Autodesk Inventor part; units mm, degrees
ref_plane "to_body_XY" through (0, 0, 0) normal (0, 1, 0) x (1, 0, 0)
ref_plane "to_body_YZ" through (0, 0, 0) normal (1, 0, 0) x (0, 0, -1)
ref_plane "to_body_ZX" through (0, 0, 0) normal (0, 0, -1) x (0, 1, 0)
sketch "Sketch_1" plane through (0, 0, 0) normal (0, 1, 0) x (-1, 0, 0)
  line L0 (3.9497, -6.3754) -> (3.9497, 6.3754)
  arc A0 (3.9497, 6.3754) -> (3.8227, 6.5024) centre (3.8227, 6.3754) ccw
  line L1 (3.8227, 6.5024) -> (-3.8227, 6.5024)
  arc A1 (-3.8227, 6.5024) -> (-3.9497, 6.3754) centre (-3.8227, 6.3754) ccw
  line L2 (-3.9497, 6.3754) -> (-3.9497, -6.3754)
  arc A2 (-3.9497, -6.3754) -> (-3.8227, -6.5024) centre (-3.8227, -6.3754) ccw
  line L3 (-3.8227, -6.5024) -> (3.8227, -6.5024)
  arc A3 (3.8227, -6.5024) -> (3.9497, -6.3754) centre (3.8227, -6.3754) ccw
  line L4 (3.6957, -6.2484) -> (3.6957, 6.2484)
  line L5 (3.6957, 6.2484) -> (-3.6957, 6.2484)
  line L6 (-3.6957, 6.2484) -> (-3.6957, -6.2484)
  line L7 (-3.6957, -6.2484) -> (3.6957, -6.2484)
extrude "Extrusion1" add sketch "Sketch_1" against normal blind 3.5814
sketch "Sketch_2" plane through (0, 0, 0) normal (0, 1, 0) x (-1, 0, 0)
  line L0 (3.9497, -6.3754) -> (3.9497, 6.3754)
  arc A0 (3.9497, 6.3754) -> (3.8227, 6.5024) centre (3.8227, 6.3754) ccw
  line L1 (3.8227, 6.5024) -> (-3.8227, 6.5024)
  arc A1 (-3.8227, 6.5024) -> (-3.9497, 6.3754) centre (-3.8227, 6.3754) ccw
  line L2 (-3.9497, 6.3754) -> (-3.9497, -6.3754)
  arc A2 (-3.9497, -6.3754) -> (-3.8227, -6.5024) centre (-3.8227, -6.3754) ccw
  line L3 (-3.8227, -6.5024) -> (3.8227, -6.5024)
  arc A3 (3.8227, -6.5024) -> (3.9497, -6.3754) centre (3.8227, -6.3754) ccw
extrude "Extrusion2" add sketch "Sketch_2" along normal blind 0.254
sketch "Sketch_7" plane through (0, 0, 0) normal (0, 0, 1) x (1, 0, 0)
  line L0 (-3.9497, 0.4023) -> (-3.9497, 0.127)
  arc A0 (-3.8227, 0.254) -> (-3.9497, 0.127) centre (-3.8227, 0.127) ccw
  line L1 (-3.8227, 0.254) -> (3.8227, 0.254)
  arc A1 (3.9497, 0.127) -> (3.8227, 0.254) centre (3.8227, 0.127) ccw
  line L2 (3.9497, 0.127) -> (3.9497, 0.4023)
  line L3 (3.9497, 0.4023) -> (-3.9497, 0.4023)
extrude "Extrusion3" cut sketch "Sketch_7" along normal mid plane 15.24
sketch "Sketch_8" plane through (0, 0, 0) normal (1, 0, 0) x (0, 1, 0)
  line L0 (0.4023, 6.5024) -> (0.127, 6.5024)
  arc A0 (0.254, 6.3754) -> (0.127, 6.5024) centre (0.127, 6.3754) ccw
  line L1 (0.254, 6.3754) -> (0.254, -6.3754)
  arc A1 (0.127, -6.5024) -> (0.254, -6.3754) centre (0.127, -6.3754) ccw
  line L2 (0.127, -6.5024) -> (0.4023, -6.5024)
  line L3 (0.4023, -6.5024) -> (0.4023, 6.5024)
extrude "Extrusion4" cut sketch "Sketch_8" along normal mid plane 15.24
sketch "Sketch_13" plane through (0, 0, 0) normal (1, 0, 0) x (0, 1, 0)
  line L0 (-3.5814, 5.08) -> (-9.4403, 5.08)
  arc A0 (-9.4403, 5.08) -> (-9.9483, 4.572) centre (-9.4403, 4.572) ccw
  line L1 (-9.9483, 4.572) -> (-9.9483, 3.2258)
  arc A1 (-10.4563, 2.7178) -> (-9.9483, 3.2258) centre (-10.4563, 3.2258) ccw
  line L2 (-10.4563, 2.7178) -> (-10.7103, 2.7178)
  line L3 (-10.7103, 2.7178) -> (-10.7103, 1.9558)
  line L4 (-10.7103, 1.9558) -> (-10.4563, 1.9558)
  arc A2 (-9.9483, 1.4478) -> (-10.4563, 1.9558) centre (-10.4563, 1.4478) ccw
  line L5 (-9.9483, 1.4478) -> (-9.9483, -1.4478)
  arc A3 (-10.4563, -1.9558) -> (-9.9483, -1.4478) centre (-10.4563, -1.4478) ccw
  line L6 (-10.4563, -1.9558) -> (-10.7103, -1.9558)
  line L7 (-10.7103, -1.9558) -> (-10.7103, -2.7178)
  line L8 (-10.7103, -2.7178) -> (-10.4563, -2.7178)
  arc A4 (-9.9483, -3.2258) -> (-10.4563, -2.7178) centre (-10.4563, -3.2258) ccw
  line L9 (-9.9483, -3.2258) -> (-9.9483, -4.572)
  arc A5 (-9.9483, -4.572) -> (-9.4403, -5.08) centre (-9.4403, -4.572) ccw
  line L10 (-9.4403, -5.08) -> (-3.5814, -5.08)
  line L11 (-3.5814, -5.08) -> (-3.5814, 5.08)
extrude "Extrusion5" add sketch "Sketch_13" along normal mid plane 7.8994
sketch "Sketch_14" plane through (0, 0, 0) normal (0, 0, 1) x (1, 0, 0)
  line L0 (-3.9497, -11.1282) -> (3.9497, -11.1282)
  line L1 (3.9497, -11.1282) -> (3.9497, -10.4563)
  arc A0 (3.6957, -10.7103) -> (3.9497, -10.4563) centre (3.6957, -10.4563) ccw
  line L2 (3.6957, -10.7103) -> (3.3147, -10.7103)
  line L3 (3.3147, -10.7103) -> (3.3147, -10.4563)
  line L4 (3.3147, -10.4563) -> (3.6322, -10.4563)
  arc A1 (3.6322, -10.4563) -> (3.6957, -10.3928) centre (3.6322, -10.3928) ccw
  line L5 (3.6957, -10.3928) -> (3.6957, -3.5814)
  line L6 (3.6957, -3.5814) -> (-3.6957, -3.5814)
  line L7 (-3.6957, -3.5814) -> (-3.6957, -10.3928)
  arc A2 (-3.6957, -10.3928) -> (-3.6322, -10.4563) centre (-3.6322, -10.3928) ccw
  line L8 (-3.6322, -10.4563) -> (-3.3147, -10.4563)
  line L9 (-3.3147, -10.4563) -> (-3.3147, -10.7103)
  line L10 (-3.3147, -10.7103) -> (-3.6957, -10.7103)
  arc A3 (-3.9497, -10.4563) -> (-3.6957, -10.7103) centre (-3.6957, -10.4563) ccw
  line L11 (-3.9497, -10.4563) -> (-3.9497, -11.1282)
extrude "Extrusion6" cut sketch "Sketch_14" along normal mid plane 10.287
sketch "Sketch_29" plane through (-3.6957, -10.7103, 1.9558) normal (0, -1, 0) x (1, 0, 0)
  line L0 (0, 0.762) -> (0, 0)
  line L1 (0, 0) -> (0.381, 0)
  arc A0 (0.381, 0) -> (0.381, 0.762) centre (0.381, 0.381) ccw
  line L2 (0.381, 0.762) -> (0, 0.762)
extrude "Extrusion7" add sketch "Sketch_29" against normal blind 0.254
sketch "Sketch_30" plane through (-3.6957, -10.7103, 1.9558) normal (0, -1, 0) x (1, 0, 0)
  arc A0 (7.0104, 0.762) -> (7.0104, 0) centre (7.0104, 0.381) ccw
  line L0 (7.0104, 0) -> (7.3914, 0)
  line L1 (7.3914, 0) -> (7.3914, 0.762)
  line L2 (7.3914, 0.762) -> (7.0104, 0.762)
extrude "Extrusion8" add sketch "Sketch_30" against normal blind 0.254
sketch "Sketch_31" plane through (-3.6957, -10.7103, -2.7178) normal (0, -1, 0) x (1, 0, 0)
  line L0 (0, 0.762) -> (0, 0)
  line L1 (0, 0) -> (0.381, 0)
  arc A0 (0.381, 0) -> (0.381, 0.762) centre (0.381, 0.381) ccw
  line L2 (0.381, 0.762) -> (0, 0.762)
extrude "Extrusion9" add sketch "Sketch_31" against normal blind 0.254
sketch "Sketch_32" plane through (-3.6957, -10.7103, -2.7178) normal (0, -1, 0) x (1, 0, 0)
  arc A0 (7.0104, 0.762) -> (7.0104, 0) centre (7.0104, 0.381) ccw
  line L0 (7.0104, 0) -> (7.3914, 0)
  line L1 (7.3914, 0) -> (7.3914, 0.762)
  line L2 (7.3914, 0.762) -> (7.0104, 0.762)
extrude "Extrusion10" add sketch "Sketch_32" against normal blind 0.254
ref_plane "to_body_XY" through (0, 0, 0) normal (0, 1, 0) x (1, 0, 0)
ref_plane "to_body_YZ" through (0, 0, 0) normal (1, 0, 0) x (0, 0, -1)
ref_plane "to_body_ZX" through (0, 0, 0) normal (0, 0, -1) x (0, 1, 0)
ref_plane "to_bushings_XY" through (0, 0.254, 0) normal (0, -1, 0) x (1, 0, 0)
ref_plane "to_bushings_YZ" through (0, 0.254, 0) normal (1, 0, 0) x (0, 0, 1)
ref_plane "to_bushings_ZX" through (0, 0.254, 0) normal (0, 0, 1) x (0, -1, 0)
properties part number "MB2011c"
Design review of the part built by this model. Coordinates are the model's own, in mm. A direction names the side the tool comes from. Coordinates: 2 decimals unless noted, no trailing zeros. Loops run counter-clockwise (first coordinate to the right, second up) from the corner with the lowest first, then second, coordinate; pieces in that order, holes last. Notation, with made-up numbers: M 86,-29.75 L 142,-29.75 A14 ccw 142,-8.75 Z; hole C 55,-40 d9. An arc over 180 degrees is marked long. Use one line per item in the form item = value.
(1) Draft analysis for pull direction X (two halves, no side actions). For faces 1 (the face through (0, -2, 6.502)), 2 (the face through (3.95, -5, 0)), 3 (the face through (0, -2, -6.248)), state which applies: pulls with the +X half, pulls with the -X half, needs draft (parallel to the pull), parting line crosses it, or undercut.
Return value:
face_1 = needs draft
face_2 = pulls with the +X half
face_3 = undercut
(2) For faces 4 (the face through (-3.95, -5, 0)), 5 (the face through (-3.696, -5, 0)), 6 (the face through (0, -2, 6.248)), list the 3-axis set-ups (+Z, -Z, +X, -X, +Y, -Y) from which the entire face can be reached by the end or side of a thin tool; tool diameter is ignored.
Return value:
face_4 = +Z, -Z, -X, +Y, -Y
face_5 = none
face_6 = -Y
(3) Consider section A-A (y = -7.5). Write out the cut boundary in (x, z).
Return value:
outline = M -3.95,-5.08 L -3.7,-5.08 L -3.7,5.08 L -3.95,5.08 Z; M 3.7,-5.08 L 3.95,-5.08 L 3.95,5.08 L 3.7,5.08 Z
(4) Consider section D-D (x = -2). Write out the cut boundary in (y, z).
Return value:
outline = M -3.58,-6.5 L 0.13,-6.5 A0.13 ccw 0.25,-6.38 L 0.25,6.38 A0.13 ccw 0.13,6.5 L -3.58,6.5 L -3.58,6.25 L 0,6.25 L 0,-6.25 L -3.58,-6.25 Z
(5) Consider section C-C (y = -2). Write out the cut boundary in (x, z), and give its area (3 significant figures).
Return value:
outline = M -3.95,-6.38 A0.13 ccw -3.82,-6.5 L 3.82,-6.5 A0.13 ccw 3.95,-6.38 L 3.95,6.38 A0.13 ccw 3.82,6.5 L -3.82,6.5 A0.13 ccw -3.95,6.38 Z; hole M -3.7,-6.25 L 3.7,-6.25 L 3.7,6.25 L -3.7,6.25 Z
area = 10.3 mm2
(6) Clearance check with flat-ended pins moving along their axes: P1, Ø1, axis at x = 2, z = 0.5, coming from the -Y side; P2, Ø4, axis at x = -2, y = -6.5, coming from the -Z side. State where each tip first meets the part, or that it passes through.
Return value:
P1 = 0
P2 = -5.08
(7) For line 1 along X through (y, z) = (-4.5, -0.25); line 2 along Z through (x, y) = (-0.5, -0.5); line 3 along Y through (x, z) = (-2, -5.5), list the stretches that pass through material, from the lowest coordinate up. Write a range as from..to.
Return value:
line_1 = -3.95..-3.7, 3.7..3.95
line_2 = -6.5..-6.25, 6.25..6.5
line_3 = 0..0.25
(8) Consider section B-B (z = 5.25). Write out the cut boundary in (x, y).
Return value:
outline = M -3.95,-3.58 L -3.7,-3.58 L -3.7,0 L 3.7,0 L 3.7,-3.58 L 3.95,-3.58 L 3.95,0.13 A0.13 ccw 3.82,0.25 L -3.82,0.25 A0.13 ccw -3.95,0.13 Z
